Verification items for the finished model (mm, model axes). Give positions to 0.01 mm unless a question says otherwise; leave off trailing zeros. Loops run counter-clockwise (first coordinate to the right, second up) from the corner with the lowest first, then second, coordinate; pieces in that order, holes last. Notation, with made-up numbers: M 84,36.25 L 102,36.25 A12 cw 102,51.25 Z; hole C 39,10 d10. An arc over 180 degrees is marked long. Answer in a Markdown table with one row per item.
```python
from build123d import *

# Parameters (mm, degrees)
SKETCH_1_R          = 1.5
SKETCH_1_R_2        = 13.5
EXTRUDE_1_DEPTH     = 5
SKETCH_2_R          = 2
CUT_EXTRUDE_1_DEPTH = 6


with BuildPart() as part:
    # 草图1 → 凸台-拉伸1 (new body)
    with BuildSketch(Plane.XY):
        with BuildLine():
            Line((-22, 0), (22, 0))
            Line((22, 0), (22, 50))
            ThreePointArc((22, 50), (0, 72), (-22, 50))
            Line((-22, 50), (-22, 0))
        make_face()
        with Locations((-15, 14)):
            Circle(SKETCH_1_R, mode=Mode.SUBTRACT)
        with Locations((-15, 4)):
            Circle(SKETCH_1_R, mode=Mode.SUBTRACT)
        with Locations((15, 4)):
            Circle(SKETCH_1_R, mode=Mode.SUBTRACT)
        with Locations((15, 14)):
            Circle(SKETCH_1_R, mode=Mode.SUBTRACT)
        with Locations((0, 50)):
            Circle(SKETCH_1_R_2, mode=Mode.SUBTRACT)
    extrude(amount=EXTRUDE_1_DEPTH)

    # 草图2 → 切除-拉伸1 (cut, through all)
    with BuildSketch(Plane(origin=(0, 0, 0), x_dir=(-1, 0, 0), z_dir=(0, 0, -1))):
        with Locations((12.374368671, 62.374368671)):
            Circle(SKETCH_2_R)
        with Locations((12.374368671, 37.625631329)):
            Circle(SKETCH_2_R)
        with Locations((-12.374368671, 37.625631329)):
            Circle(SKETCH_2_R)
        with Locations((-12.374368671, 62.374368671)):
            Circle(SKETCH_2_R)
    extrude(amount=-CUT_EXTRUDE_1_DEPTH, mode=Mode.SUBTRACT)


solid = part.part
```
Item 1: Sectioned sample at D-D (y = 55). Record the cut outline in (x, z), and give its area (3 significant figures).
Reported:
| item | result |
|---|---|
| outline | M -21.42,0 L -12.54,0 L -12.54,5 L -21.42,5 Z; M 12.54,0 L 21.42,0 L 21.42,5 L 12.54,5 Z |
| area | 88.8 mm^2 |
Item 2: Scan lines: L1, parallel to Y at x = -0.5, z = 4.5; L2, parallel to Y at x = -16, z = 4.4; L3, parallel to Y at x = 11.5, z = 2 (3 decimals). Record each from-to range of solid material in increasing order. Write a range as [from, to].
Reported:
| item | result |
|---|---|
| L1 | y = [0, 36.51], [63.49, 71.99] |
| L2 | y = [0, 2.88], [5.12, 12.88], [15.12, 65.1] |
| L3 | y = [0, 35.827], [39.424, 42.929], [57.071, 60.576], [64.173, 68.755] |
Item 3: Go/stop test with flat-tipped pins: pin 1 (1.5 mm diameter, centred on y = 62.5, z = 3, fed in from +X); pin 2 (5 mm diameter, centred on x = -12.37, y = 62.37, fed in from -Z). Record where each tip stops, or that it passes through.
Reported:
| item | result |
|---|---|
| pin 1 | stops at x = 18.6 |
| pin 2 | stops at z = 0 |
Item 4: Sectioned sample at A-A (x = 0). Record the cut outline in (y, z), and give its area (3 significant figures).
Reported:
| item | result |
|---|---|
| outline | M 0,0 L 36.5,0 L 36.5,5 L 0,5 Z; M 63.5,0 L 72,0 L 72,5 L 63.5,5 Z |
| area | 225 mm^2 |
Item 5: Sectioned sample at B-B (y = 4). Record the cut outline in (x, z).
Reported:
| item | result |
|---|---|
| outline | M -22,0 L -16.5,0 L -16.5,5 L -22,5 Z; M -13.5,0 L 13.5,0 L 13.5,5 L -13.5,5 Z; M 16.5,0 L 22,0 L 22,5 L 16.5,5 Z |
Item 6: Release check for a two-part mould opening along Y. For faces 1 (the cylindrical face through (12.808, 60.422, 2.465)), 2 (the flat face through (0, 0, 2)), 3 (the cylindrical face through (-13.297, 35.851, 2.465)), 4 (the cylindrical face through (0, 72, 2)) record: released by +Y, released by -Y, zero draft, split by the parting line, or undercut.
Reported:
| item | result |
|---|---|
| face 1 | undercut |
| face 2 | released by -Y |
| face 3 | undercut |
| face 4 | released by +Y |
Item 7: Sectioned sample at C-C (z = 2.55). State how many separate pieces and enclosed holes the cut face has, and give its area (3 significant figures).
Reported:
| item | result |
|---|---|
| separate pieces | 1 |
| enclosed holes | 9 |
| area | 2,310 mm^2 |
